Work out the finished part from the listing and answer in its coordinate system (mm). A direction names the side the tool comes from. Give positions to 0.01 mm unless a question says otherwise; leave off trailing zeros. Loops run counter-clockwise (first coordinate to the right, second up) from the corner with the lowest first, then second, coordinate; pieces in that order, holes last. Notation, with made-up numbers: (47.25, 43) - (58.25, 43) arc R18 ccw to (58.25, 60) - close; hole circle Ø3 at (63.25, -8). An arc over 180 degrees is marked (long way). One line per question, with ' | ' between items.
from build123d import *

# Parameters (mm, degrees)
BASE_EXTRUDE_DEPTH = 203.2
LSLOT_DEPTH        = 219.410047505
LPATTERN1_COUNT    = 2
LPATTERN1_PITCH    = 101.6


with BuildPart() as part:
    # Sketch1 → Base-Extrude (new body)
    with BuildSketch(Plane.XY):
        with BuildLine():
            Line((-20.6375, 18.4785), (-20.6375, -15.3416))
            ThreePointArc((-20.6375, -15.3416), (-19.848914298, -17.245414298), (-17.9451, -18.034))
            Line((-17.9451, -18.034), (17.9451, -18.034))
            ThreePointArc((17.9451, -18.034), (19.848914298, -17.245414298), (20.6375, -15.3416))
            Line((20.6375, -15.3416), (20.6375, 18.4785))
            ThreePointArc((20.6375, 18.4785), (15.875, 23.241), (11.1125, 18.4785))
            Line((11.1125, 18.4785), (11.1125, 17.44345))
            ThreePointArc((11.1125, 17.44345), (12.4587, 16.09725), (13.8049, 17.44345))
            Line((13.8049, 17.44345), (13.8049, 18.4785))
            ThreePointArc((13.8049, 18.4785), (15.875, 20.5486), (17.9451, 18.4785))
            Line((17.9451, 18.4785), (17.9451, -15.3416))
            Line((17.9451, -15.3416), (-17.9451, -15.3416))
            Line((-17.9451, -15.3416), (-17.9451, 18.4785))
            ThreePointArc((-17.9451, 18.4785), (-15.875, 20.5486), (-13.8049, 18.4785))
            Line((-13.8049, 18.4785), (-13.8049, 17.44345))
            ThreePointArc((-13.8049, 17.44345), (-12.4587, 16.09725), (-11.1125, 17.44345))
            Line((-11.1125, 17.44345), (-11.1125, 18.4785))
            ThreePointArc((-11.1125, 18.4785), (-15.875, 23.241), (-20.6375, 18.4785))
        make_face()
    extrude(amount=BASE_EXTRUDE_DEPTH)

    # Sketch2 → LSlot (cut, through all)
    with BuildSketch(Plane(origin=(1.308314937, -18.034, -10.148785872), x_dir=(1, 0, 0), z_dir=(0, -1, 0))):
        with BuildLine():
            Line((3.851060063, 88.730035872), (3.851060063, 22.848785872))
            ThreePointArc((3.851060063, 22.848785872), (-1.308314937, 17.689410872), (-6.467689937, 22.848785872))
            Line((-6.467689937, 22.848785872), (-6.467689937, 88.730035872))
            ThreePointArc((-6.467689937, 88.730035872), (-1.308314937, 93.889410872), (3.851060063, 88.730035872))
        make_face()
    lslot = extrude(amount=-LSLOT_DEPTH, mode=Mode.SUBTRACT)

    # LPattern1: LSlot ×2
    with Locations(*[(0, 0, i * LPATTERN1_PITCH) for i in range(1, LPATTERN1_COUNT)]):
        add(lslot, mode=Mode.SUBTRACT)


solid = part.part
1. Find section D-D on x = 15.5. Write down the section's boundary in (y, z).
Evaluation:
outline: (-18.03, 0) - (-15.34, 0) - (-15.34, 203.2) - (-18.03, 203.2) - close; (20.51, 0) - (23.23, 0) - (23.23, 203.2) - (20.51, 203.2) - close
2. Which of the six approach directions +Z, -Z, +X, -X, +Y, -Y give full straight-line access (tool end or side, diameter ignored) to faces 4 (the cylindrical face through (-15.77, 23.24, 100.18)), 5 (the cylindrical face through (-15.92, 20.55, 100.18)), 6 (the cylindrical face through (0.11, -16.71, 7.54))?
Evaluation:
face 4: +Z, -Z, +Y | face 5: +Z, -Z | face 6: +Y, -Y
3. Find section C-C on y = 8. Write down the section's boundary in (x, z).
Evaluation:
outline: (-20.64, 0) - (-17.95, 0) - (-17.95, 203.2) - (-20.64, 203.2) - close; (17.95, 0) - (20.64, 0) - (20.64, 203.2) - (17.95, 203.2) - close
4. Consider L1, parallel to X at y = -5, z = 34.5; L2, parallel to Y at x = 17, z = 190; L3, parallel to Y at x = 16, z = 88. Determine where each line is inside the solid, lowest interval first.
Evaluation:
L1: -20.64 to -17.95, 17.95 to 20.64 | L2: -18.03 to -15.34, 20.22 to 23.11 | L3: -18.03 to -15.34, 20.54 to 23.24
5. Find section A-A on x = 0. Write down the section's boundary in (y, z).
Evaluation:
outline: (-18.03, 0) - (-15.34, 0) - (-15.34, 7.54) - (-18.03, 7.54) - close; (-18.03, 83.74) - (-15.34, 83.74) - (-15.34, 109.14) - (-18.03, 109.14) - close; (-18.03, 185.34) - (-15.34, 185.34) - (-15.34, 203.2) - (-18.03, 203.2) - close
6. Find section B-B on z = 148. Write down the section's boundary in (x, y) (1 decimal).
Evaluation:
outline: (-20.6, -15.3) arc R2.7 ccw to (-17.9, -18) - (-5.2, -18) - (-5.2, -15.3) - (-17.9, -15.3) - (-17.9, 18.5) arc R2.1 cw to (-13.8, 18.5) - (-13.8, 17.4) arc R1.3 ccw to (-11.1, 17.4) - (-11.1, 18.5) arc R4.8 ccw to (-20.6, 18.5) - close; (5.2, -18) - (17.9, -18) arc R2.7 ccw to (20.6, -15.3) - (20.6, 18.5) arc R4.8 ccw to (11.1, 18.5) - (11.1, 17.4) arc R1.3 ccw to (13.8, 17.4) - (13.8, 18.5) arc R2.1 cw to (17.9, 18.5) - (17.9, -15.3) - (5.2, -15.3) - close
7. Determine the mould class of faces 1 (the flat face through (0, -16, 203.2)), 2 (the flat face through (20.638, 1, 100)), 3 (the cylindrical face through (-0.11, -16.71, 83.74)) for opening direction Z: +Z half, -Z half, draft (parallel to the pull), parting line (faces both ways), or undercut.
Evaluation:
face 1: +Z half | face 2: draft | face 3: undercut
8. Flat-ended cylindrical pins translate along their axes: pin 1 (0.8 mm diameter, centred on y = -17, z = 149.5, fed in from -X); pin 2 (1.3 mm diameter, centred on y = -17.5, z = 53.5, fed in from -X); pin 3 (0.8 mm diameter, centred on y = -16, z = 162.5, fed in from +X); pin 4 (1.5 mm diameter, centred on x = 16, y = -2.5, fed in from +Z). Find the tip coordinate at first contact, or state that the pin passes through.
Evaluation:
pin 1: x = -20.33 | pin 2: x = -20.18 | pin 3: x = 20.63 | pin 4: through
